Input: part model. Units: mm. Frame: model coordinates. A direction names the side the tool comes from. Round coordinates to 2 decimals unless told otherwise and drop trailing zeros. Loops run counter-clockwise (first coordinate to the right, second up) from the corner with the lowest first, then second, coordinate; pieces in that order, holes last. Notation, with made-up numbers: M 60,7.25 L 102,7.25 A31 ccw 102,38.25 Z; hole C 39.25,39 d10. An arc over 180 degrees is marked long. Use one line per item in the form item = value. Start each with the question number.
Q1. Section query B-B, the plane x = 0. Output: boundary loops of the cut face in (y, z), and give its area (4 significant figures).
Q2. Section query A-A, the plane y = 0. Output: boundary loops of the cut face in (x, z), and give its area (3 significant figures).
Q3. Mould query, pull axis X, two halves, no side actions, for faces 1 (the cylindrical face through (-1.5, 0.07, 4.94)), 2 (the conical face through (1.14, -0.02, 9.86)), 3 (the flat face through (0, 0, 9)). Classes: pulls with the +X half, pulls with the -X half, needs draft (parallel to the pull), parting line crosses it, or undercut.
Q4. Section query C-C, the plane z = 6.75. Output: boundary loops of the cut face in (x, y).
Q5. Access query for faces 4 (the flat face through (-0.5, 0, 9.5)), 5 (the flat face through (0, 0, 0)). Directions: +Z, -Z, +X, -X, +Y, -Y. A direction counts if a zero-diameter tool reaches every point of the face in a straight line with its end or side. Return the directions, or none.
Q6. Ray query, line 1 along X through (y, z) = (-0.5, 2.25); line 2 along Z through (x, y) = (-0.1, 0.65); line 3 along X through (y, z) = (0.25, 9.25). Return the intervals inside material, ascending.
```python
from build123d import *

# Parameters (mm, degrees)
SKETCH1_R           = 1.5
BOSS_EXTRUDE1_DEPTH = 10
CHAMFER1_SIZE       = 0.5
CUT_EXTRUDE1_START  = -1
CUT_EXTRUDE1_DEPTH  = 1


with BuildPart() as part:
    # Sketch1 → Boss-Extrude1 (new body)
    with BuildSketch(Plane.XY):
        Circle(SKETCH1_R)
    extrude(amount=BOSS_EXTRUDE1_DEPTH)

    # Chamfer1
    chamfer1_edges = [part.edges().sort_by_distance(p)[0] for p in [
        (-1.5, 0, 0),
        (-1.5, 0, 10),
    ]]
    chamfer(chamfer1_edges, length=CHAMFER1_SIZE)

    # Sketch2 → Cut-Extrude1 (cut)
    with BuildSketch(Plane.XY.offset(10).offset(CUT_EXTRUDE1_START)):
        with BuildLine():
            Line((-0.5, 1.414213562), (-0.5, -1.414213562))
            ThreePointArc((-0.5, -1.414213562), (0, -1.5), (0.5, -1.414213562))
            Line((0.5, -1.414213562), (0.5, 1.414213562))
            ThreePointArc((0.5, 1.414213562), (0, 1.5), (-0.5, 1.414213562))
        make_face()
    extrude(amount=CUT_EXTRUDE1_DEPTH, mode=Mode.SUBTRACT)


solid = part.part
```
Results found:
q1.outline = M -1.5,0.5 L -1,0 L 1,0 L 1.5,0.5 L 1.5,9 L -1.5,9 Z
q1.area = 26.75 mm²
q2.outline = M -1.5,0.5 L -1,0 L 1,0 L 1.5,0.5 L 1.5,9.5 L 1,10 L 0.5,10 L 0.5,9 L -0.5,9 L -0.5,10 L -1,10 L -1.5,9.5 Z
q2.area = 28.5 mm²
q3.face_1 = parting line crosses it
q3.face_2 = pulls with the +X half
q3.face_3 = undercut
q4.outline = C 0,0 d3
q5.face_4 = +Z, +Y, -Y
q5.face_5 = -Z, +X, -X, +Y, -Y
q6.line_1 = -1.41 to 1.41
q6.line_2 = 0 to 9
q6.line_3 = -1.48 to -0.5, 0.5 to 1.48
